Build history of the part. All positions in model axes, mm. A direction names the side the tool comes from. Give positions to 0.01 mm unless a question says otherwise; leave off trailing zeros. Order: outer loops, then holes, each group sorted by start corner. A loop starts at its lowest first (then second) coordinate and runs counter-clockwise, first axis right, second up. Notation, with made-up numbers: (-16, 26) -> (8, 26) arc R22 cw to (8, 48) -> close; hole circle Ø7 at (19, 62). An arc over 180 degrees is marked (long way). One line per question, with ' | ' between items. Start each with the question number.
(1) Cut at C-C (y = 2.75). Give the cut face in (x, z), then the cut area to 3 significant figures.
(2) Cut at A-A (z = 0). Give the cut face in (x, y).
(3) Drill centre lines: L1, parallel to Z at x = -5, y = 3.05; L2, parallel to X at y = 1.1, z = 3; L3, parallel to Y at x = 6, z = 0. Where is each one in solid material? Low to high. Write a range as from..to.
(4) Which spindle directions (+Z, -Z, +X, -X, +Y, -Y) get a long thin tool onto all of the face, cutting with end or side? Do faces 4 (the face through (4.25, 2.74, -3.03)), 5 (the face through (0, 5, 6)). Say none if no direction does.
(5) Cut at D-D (y = 7.25). Give the cut face in (x, z).
(6) Pull direction Z, two halves, no side cores. Call faces 1 (the face through (-5.75, 2.74, 2.97)), 2 (the face through (0, 5, -6)), 3 (the face through (0, 11, 0)): +Z half, -Z half, draft (parallel to the pull), parting line (faces both ways), or undercut.
(7) Pin check, flat tips, straight feed: pin 1 Ø3 at (y, z) = (5.5, 0) entering from +X; pin 2 Ø4 at (y, z) = (6.5, -1.5) entering from +X. Stop position of each tip, or through.
(8) Cut at B-B (x = 3.25). Give the cut face in (y, z), then the cut area to 3 significant figures.
from build123d import *

# Parameters (mm, degrees)
SKETCH1_W                      = 20
SKETCH1_H                      = 12
BOSS_EXTRUDE1_DEPTH            = 11
F_1_5_1_5_DIAMETER_HOLE1_D     = 1.5
F_1_5_1_5_DIAMETER_HOLE1_DEPTH = 5.4
F_1_5_1_5_DIAMETER_HOLE1_TIP   = 0.450645464
SKETCH6_R                      = 2
CUT_EXTRUDE1_DEPTH             = 24.600847442
FILLET1_R                      = 0.75


with BuildPart() as part:
    # Sketch1 → Boss-Extrude1 (new body)
    with BuildSketch(Plane(origin=(0, 0, 0), x_dir=(1, 0, 0), z_dir=(0, 1, 0))):
        Rectangle(SKETCH1_W, SKETCH1_H)
    extrude(amount=BOSS_EXTRUDE1_DEPTH)

    # Ø1.5 (1.5) Diameter Hole1
    with Locations(Plane(origin=(0, 0, 0), x_dir=(-1, 0, 0), z_dir=(0, -1, 0))):
        with Locations((-5, 3), (5, -3)):
            Hole(F_1_5_1_5_DIAMETER_HOLE1_D / 2, depth=F_1_5_1_5_DIAMETER_HOLE1_DEPTH)
            with Locations((0, 0, -(F_1_5_1_5_DIAMETER_HOLE1_DEPTH + F_1_5_1_5_DIAMETER_HOLE1_TIP / 2))):  # 118° drill point
                Cone(0, F_1_5_1_5_DIAMETER_HOLE1_D / 2, F_1_5_1_5_DIAMETER_HOLE1_TIP, mode=Mode.SUBTRACT)

    # Sketch6 → Cut-Extrude1 (cut, through all)
    with BuildSketch(Plane(origin=(10, 0, 0), x_dir=(0, 0, -1), z_dir=(1, 0, 0))):
        with Locations((0, 5.5)):
            Circle(SKETCH6_R)
    extrude(amount=-CUT_EXTRUDE1_DEPTH, mode=Mode.SUBTRACT)

    # Fillet1
    fillet1_edges = [part.edges().sort_by_distance(p)[0] for p in [
        (-10, 11, 0),
        (0, 11, 6),
        (10, 11, 0),
        (0, 0, 6),
        (-10, 0, 0),
        (0, 0, -6),
        (10, 0, 0),
        (0, 11, -6),
        (10, 5.5, 6),
        (-10, 5.5, 6),
        (-10, 5.5, -6),
        (10, 5.5, -6),
    ]]
    fillet(fillet1_edges, radius=FILLET1_R)


solid = part.part
Result set:
1) outline: (-10, -5.25) arc R0.75 ccw to (-9.25, -6) -> (9.25, -6) arc R0.75 ccw to (10, -5.25) -> (10, 5.25) arc R0.75 ccw to (9.25, 6) -> (-9.25, 6) arc R0.75 ccw to (-10, 5.25) -> close; hole circle Ø1.5 at (-5, 3); hole circle Ø1.5 at (5, -3) | area: 236 mm2
2) outline: (-10, 0.75) arc R0.75 ccw to (-9.25, 0) -> (9.25, 0) arc R0.75 ccw to (10, 0.75) -> (10, 3.5) -> (-10, 3.5) -> close; (-10, 7.5) -> (10, 7.5) -> (10, 10.25) arc R0.75 ccw to (9.25, 11) -> (-9.25, 11) arc R0.75 ccw to (-10, 10.25) -> close
3) L1: z = -6..2.25, 3.75..6 | L2: x = -10..-5.75, -4.25..10 | L3: y = 0..3.5, 7.5..11
4) face 4: -Y | face 5: +Z, +X, -X, +Y, -Y
5) outline: (-10, -5.25) arc R0.75 ccw to (-9.25, -6) -> (9.25, -6) arc R0.75 ccw to (10, -5.25) -> (10, -0.97) -> (-10, -0.97) -> close; (-10, 0.97) -> (10, 0.97) -> (10, 5.25) arc R0.75 ccw to (9.25, 6) -> (-9.25, 6) arc R0.75 ccw to (-10, 5.25) -> close
6) face 1: undercut | face 2: -Z half | face 3: draft
7) pin 1: passes through | pin 2: stops at x = 10
8) outline: (0, -5.25) arc R0.75 ccw to (0.75, -6) -> (10.25, -6) arc R0.75 ccw to (11, -5.25) -> (11, 5.25) arc R0.75 ccw to (10.25, 6) -> (0.75, 6) arc R0.75 ccw to (0, 5.25) -> close; hole circle Ø4 at (5.5, 0) | area: 119 mm2
